from build123d import *

# Parameters (mm, degrees)
F1_DEPTH = 30
F2_T     = -5
F4_DEPTH = 10


with BuildPart() as f1:
    # F0 (on Top) → F1 (new body)
    with BuildSketch(Plane.XY):
        Polygon((0, 75), (0, 0), (75, 0), align=None)
    extrude(amount=F1_DEPTH)

    # F2
    f2_openings = [f1.faces().sort_by_distance(p)[0] for p in [
        (37.5, 37.5, 15),
    ]]
    offset(amount=F2_T, openings=f2_openings)

    # F3 (on face) → F4 (join)
    with BuildSketch(Plane.XY.offset(30)):
        Polygon((0, 20), (0, 0), (20, 0), align=None)
    extrude(amount=F4_DEPTH)


solid = f1.part
Could you check a few things on this model? Use its own coordinates, in mm. A direction names the side the tool comes from. Give positions to 0.01 mm unless a question says otherwise; leave off trailing zeros. Write each loop counter-clockwise with the first axis right and the second up, starting at its lowest first coordinate (ties: lowest second). Pieces come first, ordered by that corner, then holes. Notation, with made-up numbers: (48, 16) - (88, 16) arc R27 cw to (88, 48) - close; hole circle Ø11 at (53, -36). An arc over 180 degrees is marked (long way). Use CSV: the item, a comma, the result in double quotes. Start each with the question number.
Item 1: I'm going to push flat-ended pins straight in: pin 1 (1.5 mm diameter, centred on y = 20, z = 29.5, fed in from +X); pin 2 (8 mm diameter, centred on x = 26, z = 12, fed in from +Y); pin 3 (22.5 mm diameter, centred on x = 24, y = 24, fed in from +Z); pin 4 (2 mm diameter, centred on y = 21.5, z = 36, fed in from -X). Where does each tip first touch, or does it pass through?
Item 2: I want a section at A-A, the plane y = 25.5. Please give me the cut outline in (x, z).
Item 3: If I drill on line 1 along Z through (x, y) = (20, 43); line 2 along X through (y, z) = (24, 10), over which ranges is the centre line in solid material (lowest first)?
Item 4: I want a section at D-D, the plane y = 54. Please give me the cut outline in (x, z).
Item 5: I want a section at C-C, the plane z = 22.5. Please give me the cut outline in (x, y).
Item 6: For faces 1 (the face through (10, 10, 35)), 2 (the face through (0, 38, 15)), 3 (the face through (23, 24, 25)), which set-ups out of +Z, -Z, +X, -X, +Y, -Y let a thin tool reach every point of the face, with its end or its side?
Item 7: I want a section at B-B, the plane x = 7.5. Please give me the cut outline in (y, z).
Findings:
1,pin 1,"stops at x = 55.75"
1,pin 2,"stops at y = 5"
1,pin 3,"stops at z = 30"
1,pin 4,"passes through"
2,outline,"(0, 0) - (49.5, 0) - (49.5, 5) - (5, 5) - (5, 25) - (49.5, 25) - (49.5, 30) - (0, 30) - close"
3,line 1,"z = 0 to 5, 25 to 30"
3,line 2,"x = 0 to 5"
4,outline,"(0, 0) - (21, 0) - (21, 5) - (5, 5) - (5, 25) - (21, 25) - (21, 30) - (0, 30) - close"
5,outline,"(0, 0) - (75, 0) - (70, 5) - (5, 5) - (5, 70) - (0, 75) - close"
6,face 1,"+Z, +X, +Y"
6,face 2,"+Z, -Z, -X, +Y, -Y"
6,face 3,"+X, +Y"
7,outline,"(0, 0) - (67.5, 0) - (67.5, 5) - (5, 5) - (5, 25) - (67.5, 25) - (67.5, 30) - (12.5, 30) - (12.5, 40) - (0, 40) - close"
